Read the model definition and answer for the solid it produces. Units are mm, in the model's axes. A direction names the side the tool comes from. Give positions to 0.01 mm unless a question says otherwise; leave off trailing zeros. Write each loop counter-clockwise with the first axis right and the second up, starting at its lowest first coordinate (ties: lowest second). Pieces come first, ordered by that corner, then holes. Notation, with made-up numbers: (85, 32.5) -> (95, 32.5) arc R23 cw to (95, 57.5) -> close; hole circle Ø7 at (71.5, 80). An arc over 180 degrees is marked (long way). Answer as CSV lines item,"result". Start each with the question number.
1. The part is cut by section C-C, the plane y = -2.5. Determine the outline of the cut face in (x, z), and give its area (3 significant figures).
2. The part is cut by section B-B, the plane z = 13. Determine the outline of the cut face in (x, y), and give its area (3 significant figures).
3. The part is cut by section D-D, the plane z = 7.5. Determine the outline of the cut face in (x, y).
4. Given pin 1 (0.5 mm diameter, centred on y = 2, z = 1, fed in from -X); pin 2 (1 mm diameter, centred on x = -1.5, z = 12, fed in from +Y); pin 3 (1.9 mm diameter, centred on x = -3.5, z = 8, fed in from +Y); pin 4 (0.9 mm diameter, centred on y = 2.5, z = 13, fed in from +X), each flat-ended and moving along its own axis, determine where each tip first touches the part or whether it passes through.
5. For a pull along X with two mould halves and no side action, classify faces 1 (the flat face through (0, -3.1, 12)), 2 (the flat face through (0, 1, 2.9)), 3 (the flat face through (-4.68, -0.69, 7.4)) as pulls with the +X half, pulls with the -X half, needs draft (parallel to the pull), parting line crosses it, or undercut.
6. Find the intervals of material crossed by line 1 (Z direction, x = 2, y = 0.75); line 2 (Z direction, x = 0, y = -2.75); line 3 (X direction, y = -0.5, z = 3.5), in increasing order.
7. A tool of negligible diameter and unlimited length cuts with its end or side. For faces 4 (the flat face through (4.5, 0, 7)), 5 (the flat face through (-4, 1.3, 2)), 6 (the flat face through (3.6, 1.3, 12.4)), 7 (the flat face through (-2, -1.9, 5)), 8 (the flat face through (0, 1, 12.1)), from which of +Z, -Z, +X, -X, +Y, -Y can it reach the whole face along a straight path? Write none if from no direction.
8. The part is cut by section A-A, the plane x = 0. Determine the outline of the cut face in (y, z), and give its area (3 significant figures).
from build123d import *

# Parameters (mm, degrees)
BOSS_EXTRUDE1_DEPTH     = 15
SKETCH2_R               = 2.6
CUT_EXTRUDE1_DEPTH      = 18.153498186
CUT_EXTRUDE2_DEPTH      = 4.6
CUT_EXTRUDE2_DEPTH_BACK = 4.6
SKETCH6_W               = 9
SKETCH6_H               = 3.2
SKETCH7_W               = 9
SKETCH7_H               = 9.2
CUT_EXTRUDE3_DEPTH      = 17.588022904


with BuildPart() as part:
    # Sketch1 → Boss-Extrude1 (new body)
    with BuildSketch(Plane.XY):
        with BuildLine():
            Line((-4.75, 1.3), (-2.4, 1.3))
            Line((-2.4, 1.3), (-2.4, 3.1))
            Line((-2.4, 3.1), (2.4, 3.1))
            Line((2.4, 3.1), (2.4, 1.3))
            Line((2.4, 1.3), (4.75, 1.3))
            ThreePointArc((4.75, 1.3), (5.490454883, 0.802863939), (5.310642707, -0.070683586))
            Line((5.310642707, -0.070683586), (3.102410151, -2.240063447))
            ThreePointArc((3.102410151, -2.240063447), (2.135739772, -2.876705813), (1, -3.1))
            Line((1, -3.1), (-1, -3.1))
            ThreePointArc((-1, -3.1), (-2.135739772, -2.876705813), (-3.102410151, -2.240063447))
            Line((-3.102410151, -2.240063447), (-5.310642707, -0.070683586))
            ThreePointArc((-5.310642707, -0.070683586), (-5.490454883, 0.802863939), (-4.75, 1.3))
        make_face()
    extrude(amount=BOSS_EXTRUDE1_DEPTH)

    # Sketch2 → Cut-Extrude1 (cut, through all)
    with BuildSketch(Plane(origin=(0, 3.1, 0), x_dir=(1, 0, 0), z_dir=(0, 1, 0))):
        with Locations(Location((0, -7.5, 0), (0, 0, 247.380135052))):
            Circle(SKETCH2_R)
    extrude(amount=-CUT_EXTRUDE1_DEPTH, mode=Mode.SUBTRACT)

    # Sketch6 → Cut-Extrude2 (cut, two sides: drawn at the far end of the back side and taken through both)
    with BuildSketch(Plane.XY.offset(7.5).offset(-CUT_EXTRUDE2_DEPTH_BACK)):
        with Locations((0, -0.3)):
            Rectangle(SKETCH6_W, SKETCH6_H)
    extrude(amount=CUT_EXTRUDE2_DEPTH + CUT_EXTRUDE2_DEPTH_BACK, mode=Mode.SUBTRACT)

    # Sketch7 → Cut-Extrude3 (cut, through all)
    with BuildSketch(Plane(origin=(0, 1.3, 0), x_dir=(1, 0, 0), z_dir=(0, 1, 0))):
        with Locations((0, -7.5)):
            Rectangle(SKETCH7_W, SKETCH7_H)
    extrude(amount=CUT_EXTRUDE3_DEPTH, mode=Mode.SUBTRACT)


solid = part.part
Results found:
1,outline,"(-2.8, 0) -> (2.8, 0) -> (2.8, 15) -> (-2.8, 15) -> close; hole circle Ø5.2 at (0, 7.5)"
1,area,"62.8 mm²"
2,outline,"(-5.31, -0.07) -> (-3.1, -2.24) arc R3 ccw to (-1, -3.1) -> (1, -3.1) arc R3 ccw to (3.1, -2.24) -> (5.31, -0.07) arc R0.8 ccw to (4.75, 1.3) -> (2.4, 1.3) -> (2.4, 3.1) -> (-2.4, 3.1) -> (-2.4, 1.3) -> (-4.75, 1.3) arc R0.8 ccw to start"
2,area,"46.0 mm²"
3,outline,"(-5.31, -0.07) -> (-4.5, -0.87) -> (-4.5, 1.3) -> (-4.75, 1.3) arc R0.8 ccw to start; (-3.45, -1.9) -> (-3.1, -2.24) arc R3 ccw to (-2.6, -2.64) -> (-2.6, -1.9) -> close; (2.6, -2.64) arc R3 ccw to (3.1, -2.24) -> (3.45, -1.9) -> (2.6, -1.9) -> close; (4.5, -0.87) -> (5.31, -0.07) arc R0.8 ccw to (4.75, 1.3) -> (4.5, 1.3) -> close"
4,pin 1,"stops at x = -2.4"
4,pin 2,"stops at y = 3.1"
4,pin 3,"stops at y = -1.9"
4,pin 4,"stops at x = 2.4"
5,face 1,"needs draft"
5,face 2,"undercut"
5,face 3,"pulls with the -X half"
6,line 1,"z = 0 to 2.9, 12.1 to 15"
6,line 2,"z = 0 to 4.9, 10.1 to 15"
6,line 3,"x = -4.87 to -4.5, 4.5 to 4.87"
7,face 4,"+Y, -Y"
7,face 5,"+Z, -Z, -X, +Y"
7,face 6,"+Z, -Z, +X, +Y"
7,face 7,"+X, -X, +Y"
7,face 8,"+Y"
8,outline,"(-3.1, 0) -> (3.1, 0) -> (3.1, 2.9) -> (-1.9, 2.9) -> (-1.9, 4.9) -> (-3.1, 4.9) -> close; (-3.1, 10.1) -> (-1.9, 10.1) -> (-1.9, 12.1) -> (3.1, 12.1) -> (3.1, 15) -> (-3.1, 15) -> close"
8,area,"40.8 mm²"
